from build123d import *

# Parameters (mm, degrees)
SKETCH1_W                           = 140.716
SKETCH1_H                           = 139.7
MAIN_BODY_DEPTH                     = 3.175
SKETCH2_R                           = 24.13
CUTS_FOR_EYES_AND_MOTORS_DEPTH      = 4.175
SKETCH4_W                           = 3.2258
SKETCH4_H                           = 50.8
CUT_FOR_NOSE_DEPTH                  = 4.175
CUT_FOR_ROUNDED_FACE_FEATURES_DEPTH = 4.175
SKETCH12_R                          = 1.524
HOLES_FOR_SPACERS_DEPTH             = 4.175
BOSS_EXTRUDE1_DEPTH                 = 3.175


with BuildPart() as part:
    # Sketch1 → main body (new body)
    with BuildSketch(Plane.XY):
        with Locations((0, -69.85)):
            Rectangle(SKETCH1_W, SKETCH1_H)
    extrude(amount=MAIN_BODY_DEPTH)

    # Sketch2 → cuts for eyes and motors (cut, through all)
    with BuildSketch(Plane.XY.offset(3.175)):
        with Locations((-33.528, -48.26)):
            Circle(SKETCH2_R)
    cuts_for_eyes_and_motors = extrude(amount=-CUTS_FOR_EYES_AND_MOTORS_DEPTH, mode=Mode.SUBTRACT)

    # Sketch4 → cut for nose (cut, through all)
    with BuildSketch(Plane.XY.offset(3.175)):
        with Locations((0, -82.55)):
            Rectangle(SKETCH4_W, SKETCH4_H)
    extrude(amount=-CUT_FOR_NOSE_DEPTH, mode=Mode.SUBTRACT)

    # Mirror1: cuts for eyes and motors across plane
    add(cuts_for_eyes_and_motors.mirror(Plane(origin=(0, 0, 0), x_dir=(0, 0, 1), z_dir=(1, 0, 0))), mode=Mode.SUBTRACT)

    # Sketch11 → cut for rounded face features (cut, through all)
    with BuildSketch(Plane.XY.offset(3.175)):
        with BuildLine():
            Line((-70.358, -139.7), (-70.358, -86.36))
            ThreePointArc((-70.358, -86.36), (-55.943359781, -111.56490753), (-48.768, -139.7))
            Line((-48.768, -139.7), (-70.358, -139.7))
        make_face()
        with BuildLine():
            Line((-70.358, 0), (-70.358, -13.97))
            ThreePointArc((-70.358, -13.97), (-64.724440046, -5.321180316), (-55.88, 0))
            Line((-55.88, 0), (-70.358, 0))
        make_face()
    cut_for_rounded_face_features = extrude(amount=-CUT_FOR_ROUNDED_FACE_FEATURES_DEPTH, mode=Mode.SUBTRACT)

    # mirror of rounded feature: cut for rounded face features across plane
    add(cut_for_rounded_face_features.mirror(Plane(origin=(0, 0, 0), x_dir=(0, 0, 1), z_dir=(1, 0, 0))), mode=Mode.SUBTRACT)

    # Sketch12 → holes for spacers (cut, through all)
    with BuildSketch(Plane.XY.offset(3.175)):
        with Locations((-57.658, -7.62)):
            Circle(SKETCH12_R)
        with Locations((-60.198, -83.82)):
            Circle(SKETCH12_R)
        with Locations((-50.038, -114.3)):
            Circle(SKETCH12_R)
    holes_for_spacers = extrude(amount=-HOLES_FOR_SPACERS_DEPTH, mode=Mode.SUBTRACT)

    # mirror of spacer hole: holes for spacers across plane
    add(holes_for_spacers.mirror(Plane(origin=(0, 0, 0), x_dir=(0, 0, 1), z_dir=(1, 0, 0))), mode=Mode.SUBTRACT)

    # Sketch14 → Boss-Extrude1 (add)
    with BuildSketch(Plane.XY.offset(3.175)):
        Polygon((-48.768, -139.7), (-35.433, -139.7), (-35.433, -157.48), (-48.768, -151.596070028), align=None)
    boss_extrude1 = extrude(amount=-BOSS_EXTRUDE1_DEPTH)

    # Mirror3: Boss-Extrude1 across plane
    add(boss_extrude1.mirror(Plane(origin=(0, 0, 0), x_dir=(0, 0, 1), z_dir=(1, 0, 0))))


solid = part.part
Design review of the part built by this model. Coordinates are the model's own, in mm. A direction names the side the tool comes from. Coordinates: 2 decimals unless noted, no trailing zeros. Order: outer loops, then holes, each group sorted by start corner. A loop starts at its lowest first (then second) coordinate and runs counter-clockwise, first axis right, second up. Notation, with made-up numbers: (-17.5, -37.5) -> (2.5, -37.5) arc R32 ccw to (2.5, -10.5) -> close; hole circle Ø3 at (0.5, 46). An arc over 180 degrees is marked (long way). Use one line per item in the form item = value. Start each with the question number.
(1) Add section C-C on x = -46. State the section outline as (y, z) points (3 decimals), plus the area to 3 significant figures.
(2) For probe 1 along X at (y, z) = (-34, 1.7); probe 2 along X at (y, z) = (-114.3, 1.5); probe 3 along X at (y, z) = (-145.5, 1.2), list the stretches that pass through material, from the lowest coordinate up.
(3) Insertion check: pin 1 (5 mm diameter, centred on x = -60.198, y = -83.82, fed in from -Z); pin 2 (1 mm diameter, centred on y = -89, z = 2.5, fed in from +X); pin 3 (1 mm diameter, centred on x = -4.5, z = 2.5, fed in from -Y); pin 4 (1 mm diameter, centred on y = -99, z = 2, fed in from +X). Each pin has a flat end and moves straight along its axis. Give the tip position at first contact, or say it passes through.
(4) The part is to be moulded in two halves that separate along Y. For faces 5 (the flat face through (0, -139.7, 2)), 6 (the flat face through (1.613, -83, 2)), 7 (the flat face through (-17, -78, 0)), say which applies: +Y half, -Y half, draft (parallel to the pull), parting line (faces both ways), or undercut.
(5) Add section B-B on z = 0.65. Give the number of separate pieces and of enclosed holes in the cut face, plus the area to 3 significant figures.
(6) Add section A-A on y = -77. State the section outline as (x, z) points (3 decimals).
(7) For faces 1 (the flat face through (-48.768, -146, 2)), 2 (the flat face through (-35.433, -148, 2)), 3 (the flat face through (48.768, -146, 2)), 4 (the flat face through (0, -57.15, 2)), list the 3-axis set-ups (+Z, -Z, +X, -X, +Y, -Y) from which the entire face can be reached by the end or side of a thin tool; tool diameter is ignored.
(8) Add section D-D on y = -46.5. State the section outline as (x, z) points (3 decimals).
Answer block:
q1.outline = (-152.817, 0) -> (-68.917, 0) -> (-68.917, 3.175) -> (-152.817, 3.175) -> close; (-27.603, 0) -> (0, 0) -> (0, 3.175) -> (-27.603, 3.175) -> close
q1.area = 354 mm²
q2.probe_1 = -70.36 to -52.99, -14.06 to 14.06, 52.99 to 70.36
q2.probe_2 = -54.88 to -51.56, -48.51 to 48.51, 51.56 to 54.88
q2.probe_3 = -48.77 to -35.43, 35.43 to 48.77
q3.pin_1 = 0
q3.pin_2 = 68.76
q3.pin_3 = -139.7
q3.pin_4 = 62.29
q4.face_5 = -Y half
q4.face_6 = undercut
q4.face_7 = draft
q5.separate_pieces = 1
q5.enclosed_holes = 9
q5.area = 14,600 mm²
q6.outline = (-70.358, 0) -> (-1.613, 0) -> (-1.613, 3.175) -> (-70.358, 3.175) -> close; (1.613, 0) -> (70.358, 0) -> (70.358, 3.175) -> (1.613, 3.175) -> close
q7.face_1 = +Z, -Z, -X, -Y
q7.face_2 = +Z, -Z, -Y
q7.face_3 = +Z, -Z, +X, -Y
q7.face_4 = +Z, -Z
q8.outline = (-70.358, 0) -> (-57.594, 0) -> (-57.594, 3.175) -> (-70.358, 3.175) -> close; (-9.462, 0) -> (9.462, 0) -> (9.462, 3.175) -> (-9.462, 3.175) -> close; (57.594, 0) -> (70.358, 0) -> (70.358, 3.175) -> (57.594, 3.175) -> close
